Geometry: final body of the model. Coordinates: model frame, mm. A direction names the side the tool comes from. Give positions to 0.01 mm unless a question says otherwise; leave off trailing zeros. Write each loop counter-clockwise with the first axis right and the second up, starting at its lowest first coordinate (ties: lowest second). Pieces come first, ordered by that corner, then holes. Notation, with made-up numbers: M -32.5,-10.75 L 1.5,-10.75 A11 ccw 1.5,2.25 Z; hole C -37,39.25 d6. An arc over 180 degrees is marked long. Use a Markdown table: item, result. Add a question column.
1) Set-up query: faces 1 (the flat face through (-71.4, 16.5, 69.6)), 2 (the flat face through (-1, 5, 72.5)), 3 (the flat face through (71.3, 16.5, -70.3)), 4 (the flat face through (71.3, 16.5, 70.2)). Return all of +Z, -Z, +X, -X, +Y, -Y with unobstructed straight access to the full face (end or side cutting, diameter ignored); none if empty.
2) Section D-D on x = 6. Return the cut outline in (y, z).
3) Pin query (flat end, axial travel): pin 1 (3.5 mm diameter, centred on y = 18.5, z = -73.5, fed in from -X); pin 2 (2.5 mm diameter, centred on y = 18.5, z = -73.5, fed in from +X); pin 3 (2 mm diameter, centred on x = -33.5, z = -39, fed in from +Y). Return the tip coordinate at first contact, or that it passes through.
4) Section A-A on y = -9.5. Return the cut outline in (x, z).
5) Line query: line 1 (X direction, y = -14.2, z = 52); line 2 (X direction, y = -15, z = 2); line 3 (Z direction, x = -55.5, y = -4.5). Output: solid intervals per line, ascending.
6) Section C-C on y = 0. Return the cut outline in (x, z), then the cut area to 3 significant figures.
7) Section B-B on z = -31. Return the cut outline in (x, y), then the cut area to 3 significant figures.
```python
from build123d import *

# Parameters (mm, degrees)
SKETCH1_W           = 151
SKETCH1_H           = 151
BOSS_EXTRUDE1_DEPTH = 16.5
SKETCH2_W           = 145
SKETCH2_H           = 145
CUT_EXTRUDE1_DEPTH  = 30
SKETCH3_W           = 4
SKETCH3_H           = 50
CUT_EXTRUDE2_DEPTH  = 111.907619215
SKETCH6_W           = 121
SKETCH6_H           = 3
BOSS_EXTRUDE2_DEPTH = 6
SKETCH7_W           = 3
SKETCH7_H           = 121
BOSS_EXTRUDE3_DEPTH = 6
CUT_EXTRUDE3_REACH  = 172.316
SKETCH8_R           = 3
FILLET1_R           = 10
FILLET2_R           = 7
FILLET3_R           = 2.5
SKETCH12_R          = 1.5
CUT_EXTRUDE4_DEPTH  = 114.672775984


with BuildPart() as part:
    # Sketch1 → Boss-Extrude1 (new, symmetric)
    with BuildSketch(Plane(origin=(0, 0, 0), x_dir=(1, 0, 0), z_dir=(0, 1, 0))):
        Rectangle(SKETCH1_W, SKETCH1_H)
    extrude(amount=BOSS_EXTRUDE1_DEPTH, both=True)

    # Sketch2 → Cut-Extrude1 (cut)
    with BuildSketch(Plane(origin=(0, 16.5, 0), x_dir=(1, 0, 0), z_dir=(0, 1, 0))):
        Rectangle(SKETCH2_W, SKETCH2_H)
    extrude(amount=-CUT_EXTRUDE1_DEPTH, mode=Mode.SUBTRACT)

    # Sketch3 → Cut-Extrude2 (cut, through all)
    with BuildSketch(Plane(origin=(0, -13.5, 0), x_dir=(1, 0, 0), z_dir=(0, 1, 0))):
        with Locations((-65, -42)):
            Rectangle(SKETCH3_W, SKETCH3_H)
        with Locations((-65, 42)):
            Rectangle(SKETCH3_W, SKETCH3_H)
    cut_extrude2 = extrude(amount=-CUT_EXTRUDE2_DEPTH, mode=Mode.SUBTRACT)

    # Mirror1: Cut-Extrude2 across plane
    add(cut_extrude2.mirror(Plane(origin=(0, 0, 0), x_dir=(0, 0, 1), z_dir=(1, 0, 0))), mode=Mode.SUBTRACT)

    # Sketch6 → Boss-Extrude2 (add)
    with BuildSketch(Plane(origin=(0, 16.5, 0), x_dir=(1, 0, 0), z_dir=(0, 1, 0))):
        with Locations((0, -74)):
            Rectangle(SKETCH6_W, SKETCH6_H)
    boss_extrude2 = extrude(amount=BOSS_EXTRUDE2_DEPTH)

    # Mirror2: Boss-Extrude2 across plane
    add(boss_extrude2.mirror(Plane.XY))

    # Sketch7 → Boss-Extrude3 (add)
    with BuildSketch(Plane(origin=(0, 16.5, 0), x_dir=(1, 0, 0), z_dir=(0, 1, 0))):
        with Locations((-74, 0)):
            Rectangle(SKETCH7_W, SKETCH7_H)
    boss_extrude3 = extrude(amount=BOSS_EXTRUDE3_DEPTH)

    # Mirror4: Boss-Extrude3 across plane
    add(boss_extrude3.mirror(Plane(origin=(0, 0, 0), x_dir=(0, 0, 1), z_dir=(1, 0, 0))))

    # Sketch8 → Cut-Extrude3 (cut, up to next)
    with BuildSketch(Plane(origin=(75.5, 0, 0), x_dir=(0, 0, -1), z_dir=(1, 0, 0)), mode=Mode.PRIVATE) as cut_extrude3_sk1:
        Circle(SKETCH8_R)
    cut_extrude3_tool1 = extrude(cut_extrude3_sk1.sketch, amount=-CUT_EXTRUDE3_REACH, mode=Mode.PRIVATE) & part.part
    add(cut_extrude3_tool1.solids().sort_by_distance((75.5, 0, 0))[0], mode=Mode.SUBTRACT)

    # Fillet1
    fillet1_edges = [part.edges().sort_by_distance(p)[0] for p in [
        (75.5, 0, 75.5),
        (-75.5, 0, 75.5),
        (-75.5, 0, -75.5),
        (75.5, 0, -75.5),
    ]]
    fillet(fillet1_edges, radius=FILLET1_R)

    # Fillet2
    fillet2_edges = [part.edges().sort_by_distance(p)[0] for p in [
        (72.5, 1.5, -72.5),
        (72.5, 1.5, 72.5),
        (-72.5, 1.5, 72.5),
        (-72.5, 1.5, -72.5),
    ]]
    fillet(fillet2_edges, radius=FILLET2_R)

    # Fillet3
    fillet3_edges = [part.edges().sort_by_distance(p)[0] for p in [
        (-60.5, 22.5, -74),
        (60.5, 22.5, -74),
        (-74, 22.5, -60.5),
        (-74, 22.5, 60.5),
        (74, 22.5, 60.5),
        (74, 22.5, -60.5),
        (-60.5, 22.5, 74),
        (60.5, 22.5, 74),
    ]]
    fillet(fillet3_edges, radius=FILLET3_R)

    # Sketch12 → Cut-Extrude4 (cut, through all)
    with BuildSketch(Plane.XZ.offset(16.5)):
        with Locations(Location((-25, 52, 0), (0, 0, 270))):
            Circle(SKETCH12_R)
        with Locations(Location((-25, 2, 0), (0, 0, 270))):
            Circle(SKETCH12_R)
        with Locations(Location((25, 52, 0), (0, 0, 270))):
            Circle(SKETCH12_R)
        with Locations(Location((25, 2, 0), (0, 0, 270))):
            Circle(SKETCH12_R)
        with Locations(Location((-25, -48, 0), (0, 0, 270))):
            Circle(SKETCH12_R)
        with Locations(Location((25, -48, 0), (0, 0, 270))):
            Circle(SKETCH12_R)
    extrude(amount=-CUT_EXTRUDE4_DEPTH, mode=Mode.SUBTRACT)


solid = part.part
```
Found:
| question | item | result |
|---|---|---|
| 1 | face 1 | +Z, -X, +Y |
| 1 | face 2 | +Y |
| 1 | face 3 | -Z, +X, +Y |
| 1 | face 4 | +Z, +X, +Y |
| 2 | outline | M -16.5,-75.5 L 22.5,-75.5 L 22.5,-72.5 L -13.5,-72.5 L -13.5,72.5 L 22.5,72.5 L 22.5,75.5 L -16.5,75.5 Z |
| 3 | pin 1 | x = -60.5 |
| 3 | pin 2 | x = 60.5 |
| 3 | pin 3 | y = -13.5 |
| 4 | outline | M -75.5,-65.5 A10 ccw -65.5,-75.5 L 65.5,-75.5 A10 ccw 75.5,-65.5 L 75.5,65.5 A10 ccw 65.5,75.5 L -65.5,75.5 A10 ccw -75.5,65.5 Z; hole M -72.5,-65.5 A7 ccw -65.5,-72.5 L 65.5,-72.5 A7 ccw 72.5,-65.5 L 72.5,65.5 A7 ccw 65.5,72.5 L -65.5,72.5 A7 ccw -72.5,65.5 Z |
| 5 | line 1 | -75.5 to -67, -63 to -26.5, -23.5 to 23.5, 26.5 to 63, 67 to 75.5 |
| 5 | line 2 | -75.5 to -26.5, -23.5 to 23.5, 26.5 to 75.5 |
| 5 | line 3 | -75.5 to -72.5, 72.5 to 75.5 |
| 6 | outline | M -75.5,-65.5 A10 ccw -65.5,-75.5 L 65.5,-75.5 A10 ccw 75.5,-65.5 L 75.5,-3 L 72.5,-3 L 72.5,-65.5 A7 cw 65.5,-72.5 L -65.5,-72.5 A7 cw -72.5,-65.5 L -72.5,65.5 A7 cw -65.5,72.5 L 65.5,72.5 A7 cw 72.5,65.5 L 72.5,3 L 75.5,3 L 75.5,65.5 A10 ccw 65.5,75.5 L -65.5,75.5 A10 ccw -75.5,65.5 Z |
| 6 | area | 1,710 mm² |
| 7 | outline | M -75.5,-16.5 L -67,-16.5 L -67,-13.5 L -72.5,-13.5 L -72.5,22.5 L -75.5,22.5 Z; M -63,-16.5 L 63,-16.5 L 63,-13.5 L -63,-13.5 Z; M 67,-16.5 L 75.5,-16.5 L 75.5,22.5 L 72.5,22.5 L 72.5,-13.5 L 67,-13.5 Z |
| 7 | area | 645 mm² |
